The model under review builds one solid part; all positions refer to its coordinate system, in mm. Give positions to 0.01 mm unless a question says otherwise; leave off trailing zeros. Order: outer loops, then holes, each group sorted by start corner. A loop starts at its lowest first (then second) coordinate and runs counter-clockwise, first axis right, second up. Notation, with made-up numbers: (75.25, 37) - (79.25, 37) arc R28 cw to (79.25, 64) - close; hole circle Ø11 at (86.5, 11.5). An arc over 180 degrees is marked (long way). Use CSV: the item, a comma, the result in double quotes.
```python
from build123d import *

# Parameters (mm, degrees)
ESBO_O1_W                = 126
ESBO_O1_H                = 74
ESBO_O1_R                = 1.7
ESBO_O1_R_2              = 7.5
RESSALTO_EXTRUS_O1_DEPTH = 2


with BuildPart() as part:
    # Esboço1 → Ressalto-extrusão1 (new body)
    with BuildSketch(Plane.XY):
        with Locations((63, -37)):
            Rectangle(ESBO_O1_W, ESBO_O1_H)
        with Locations((47, -6)):
            Circle(ESBO_O1_R, mode=Mode.SUBTRACT)
        with Locations((109, -6)):
            Circle(ESBO_O1_R, mode=Mode.SUBTRACT)
        with Locations((47, -68)):
            Circle(ESBO_O1_R, mode=Mode.SUBTRACT)
        with Locations((109, -68)):
            Circle(ESBO_O1_R, mode=Mode.SUBTRACT)
        with Locations((25, -37)):
            Circle(ESBO_O1_R_2, mode=Mode.SUBTRACT)
        with BuildLine():
            Line((50, -3), (50, -17.712698478))
            ThreePointArc((50, -17.712698478), (44, -37), (50, -56.287301522))
            Line((50, -56.287301522), (50, -71))
            Line((50, -71), (106, -71))
            Line((106, -71), (106, -56.287301522))
            ThreePointArc((106, -56.287301522), (112, -37), (106, -17.712698478))
            Line((106, -17.712698478), (106, -3))
            Line((106, -3), (50, -3))
        make_face(mode=Mode.SUBTRACT)
    extrude(amount=RESSALTO_EXTRUS_O1_DEPTH)


solid = part.part
```
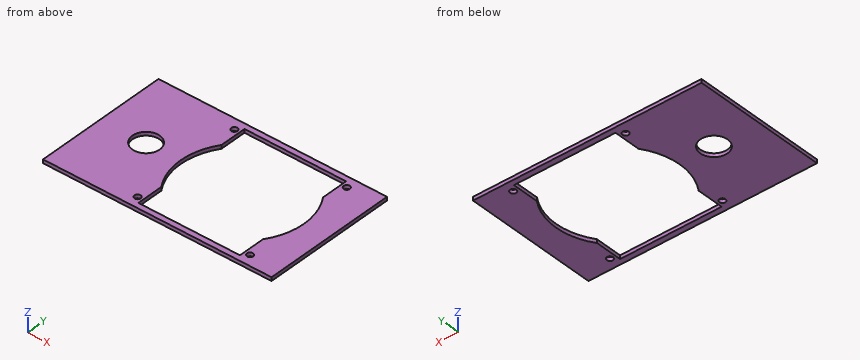
Item 1: Take a section at C-C, the plane z = 0.8. Give the boundary of the cut face in (x, y).
Results list:
outline,"(0, -74) - (126, -74) - (126, 0) - (0, 0) - close; hole circle Ø15 at (25, -37); hole circle Ø3.4 at (47, -68); hole circle Ø3.4 at (47, -6); hole (50, -71) - (106, -71) - (106, -56.29) arc R34 ccw to (106, -17.71) - (106, -3) - (50, -3) - (50, -17.71) arc R34 ccw to (50, -56.29) - close; hole circle Ø3.4 at (109, -68); hole circle Ø3.4 at (109, -6)"
Item 2: Wall thickness on L1, parallel to X at y = -68, z = 1.2; L2, parallel to Y at x = 93.5, z = 1.1; L3, parallel to X at y = -8.5, z = 0.7: over which ranges is each line inside the solid? List them lowest first.
Results list:
L1,"x = 0 to 45.3, 48.7 to 50, 106 to 107.3, 110.7 to 126"
L2,"y = -74 to -71, -3 to 0"
L3,"x = 0 to 50, 106 to 126"
Item 3: Take a section at B-B, the plane x = 25. Give the boundary of the cut face in (y, z), and give its area (3 significant figures).
Results list:
outline,"(-74, 0) - (-44.5, 0) - (-44.5, 2) - (-74, 2) - close; (-29.5, 0) - (0, 0) - (0, 2) - (-29.5, 2) - close"
area,"118 mm2"
Item 4: Clearance check with flat-ended pins moving along their axes: pin 1 (13.5 mm diameter, centred on x = 25, y = -37, fed in from +Z); pin 2 (1 mm diameter, centred on y = -11.5, z = 1, fed in from -X). State where each tip first meets the part, or that it passes through.
Results list:
pin 1,"passes through"
pin 2,"stops at x = 0"
Item 5: Take a section at A-A, the plane y = -68. Give the boundary of the cut face in (x, z), and give its area (3 significant figures).
Results list:
outline,"(0, 0) - (45.3, 0) - (45.3, 2) - (0, 2) - close; (48.7, 0) - (50, 0) - (50, 2) - (48.7, 2) - close; (106, 0) - (107.3, 0) - (107.3, 2) - (106, 2) - close; (110.7, 0) - (126, 0) - (126, 2) - (110.7, 2) - close"
area,"126 mm2"
Item 6: Take a section at D-D, the plane y = -37. Give the boundary of the cut face in (x, z), and give its area (3 significant figures).
Results list:
outline,"(0, 0) - (17.5, 0) - (17.5, 2) - (0, 2) - close; (32.5, 0) - (44, 0) - (44, 2) - (32.5, 2) - close; (112, 0) - (126, 0) - (126, 2) - (112, 2) - close"
area,"86.0 mm2"
